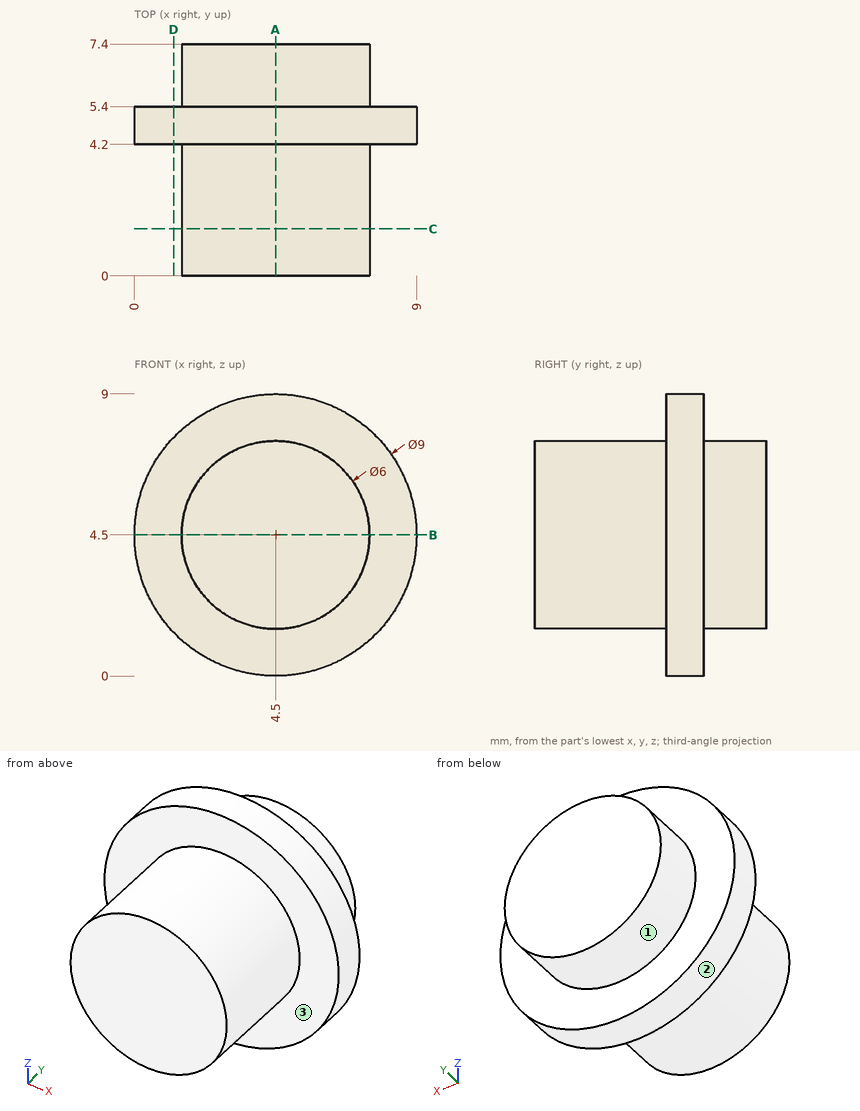
Check sheet for the drawn part. Datum: minimum x, y, z corner. Units: mm. A direction names the side the tool comes from. Give positions to 0.01 mm unless a question says otherwise; leave off trailing zeros. Loops run counter-clockwise (first coordinate to the right, second up) from the corner with the lowest first, then second, coordinate; pieces in that order, holes last.
1) Sectioned sample at D-D, the plane x = 1.25. Enter the section's corners in (y, z), then the cut area to 3 significant figures.
2) Thickness scan on line 1 along Y through (x, z) = (4.25, 1.25); line 2 along Z through (x, y) = (1.25, 4.5); line 3 along Z through (x, y) = (1.75, 2.5). Record the ranges inside material, lowest first.
3) Sectioned sample at C-C, the plane y = 1.5. Enter the section's corners in (x, z).
4) Sectioned sample at B-B, the plane z = 4.5. Enter the section's corners in (x, y).
5) Set-up check for the marked faces 1, 2 and 3: record each of +Z, -Z, +X, -X, +Y, -Y from which the full face is reachable in a straight line by a thin tool's end or side.
6) Sectioned sample at A-A, the plane x = 4.5. Enter the section's corners in (y, z), then the cut area to 3 significant figures.
7) Depth check by flat-ended pin: pin 1 Ø1 at (x, z) = (4, 7) entering from -Y; pin 2 Ø3 at (y, z) = (6.5, 2) entering from -X; pin 3 Ø2 at (x, y) = (7, 1) entering from -Z; pin 4 Ø1.5 at (y, z) = (4.5, 6) entering from -X. Enter the tip coordinate at first touch or a pass-through.
Answers:
1. outline: (4.2, 1.39) - (5.4, 1.39) - (5.4, 7.61) - (4.2, 7.61) - close
1. area: 7.47 mm2
2. line 1: y = 4.2 to 5.4
2. line 2: z = 1.39 to 7.61
2. line 3: z = 3.3 to 5.7
3. outline: circle Ø6 at (4.5, 4.5)
4. outline: (0, 4.2) - (1.5, 4.2) - (1.5, 0) - (7.5, 0) - (7.5, 4.2) - (9, 4.2) - (9, 5.4) - (7.5, 5.4) - (7.5, 7.4) - (1.5, 7.4) - (1.5, 5.4) - (0, 5.4) - close
5. face 1: +Y
5. face 2: +Y, -Y
5. face 3: -Y
6. outline: (0, 1.5) - (4.2, 1.5) - (4.2, 0) - (5.4, 0) - (5.4, 1.5) - (7.4, 1.5) - (7.4, 7.5) - (5.4, 7.5) - (5.4, 9) - (4.2, 9) - (4.2, 7.5) - (0, 7.5) - close
6. area: 48.0 mm2
7. pin 1: stops at y = 0
7. pin 2: stops at x = 0.25
7. pin 3: stops at z = 1.9
7. pin 4: stops at x = 0.06
